Autodesk Inventor part; units mm, degrees
ref_plane "Work Plane2" through (-55.1754, -24.0887, 15.745) normal (0, 0, -1) x (0, 1, 0)
ref_plane "YZ Plane" through (0, 0, 0) normal (1, 0, 0) x (0, 1, 0)
ref_plane "XZ Plane" through (0, 0, 0) normal (0, 1, 0) x (-1, 0, 0)
ref_plane "Work Plane1" through (0, 0, 0) normal (0, 0, 1) x (1, 0, 0)
ref_plane "Work Plane2" through (-55.1754, -24.0887, 15.745) normal (0, 0, -1) x (0, 1, 0)
sketch "Sketch1" plane through (0, 0, 0) normal (0, 0, 1) x (1, 0, 0)
  line L0 (-15.577, -32.8319) -> (-625.177, -32.8319)
  line L1 (-15.577, -13.7819) -> (-625.177, -13.7819)
  line L2 (-51.9475, -0.5269) -> (-51.9475, -17.8187)
  line L3 (-15.577, -10.6107) -> (-15.577, -36.0031)
  line L4 (-51.9475, -45.8894) -> (-31.9475, -45.8894)
  line L5 (-51.9475, -13.7819) -> (-9.7581, -13.7819)
  line L6 (-9.7581, -13.7819) -> (-9.7581, -45.8894)
  line L7 (-9.7581, -45.8894) -> (-51.9475, -45.8894)
  line L8 (-51.9475, -45.8894) -> (-51.9475, -13.7819)
  arc A0 (-55.86, -21.5601) -> (-54.5757, -21.9771) centre (-55.7173, -23.3069) ccw
  arc A1 (-28.9193, -21.5601) -> (-27.635, -21.9771) centre (-28.7766, -23.3069) ccw
  circle A2 centre (-55.7173, -23.3069) radius 1.778
  circle A3 centre (-28.7766, -23.3069) radius 1.778
  circle A4 centre (-37.9475, -17.22) radius 2
  circle A5 centre (-37.9475, -17.22) radius 2
  point P0 (0, 0)
extrude "Extrusion1" add sketch "Sketch1" along normal up to surface (15.745 mm away) contours L3 L5 L6 L7 L4 L8 L0 | L0 L8 L2 L1 L3 | A4
sketch "Sketch2" plane through (-51.9475, -13.7819, 15.745) normal (0, 0, 1) x (1, 0, 0)
  circle A0 centre (6, -26.745) radius 2
  circle A1 centre (14, -26.745) radius 2
  circle A2 centre (6, -26.745) radius 2
  circle A3 centre (14, -26.745) radius 2
  point P0 (51.9475, 13.7819)
hole "Hole1" at (-45.9475, -40.5269, 15.745) direction (0, 0, -1) diameter 3.9878 end through all
sketch "Sketch3" plane through (-51.9475, -13.7819, 15.745) normal (0, 0, 1) x (1, 0, 0)
  circle A0 centre (14, -26.745) radius 2
  circle A1 centre (14, -26.745) radius 2
  point P0 (51.9475, 13.7819)
hole "Hole2" at (-37.9475, -40.5269, 15.745) direction (0, 0, -1) diameter 3.9878 end through all
sketch "Sketch5" plane through (-51.9475, -13.7819, 15.745) normal (0, 0, 1) x (1, 0, 0)
  arc A0 (5.0711, -20.6445) -> (7.8995, -17.8161) centre (6.4853, -19.2303) ccw
  line L0 (4.5858, -20.1592) -> (5.0711, -20.6445)
  arc A1 (7.4142, -17.3308) -> (4.5858, -20.1592) centre (6, -18.745) ccw
  line L1 (7.8995, -17.8161) -> (7.4142, -17.3308)
  arc A2 (7.8995, -3.6739) -> (5.0711, -0.8455) centre (6.4853, -2.2597) ccw
  line L2 (7.4142, -4.1592) -> (7.8995, -3.6739)
  arc A3 (4.5858, -1.3308) -> (7.4142, -4.1592) centre (6, -2.745) ccw
  line L3 (5.0711, -0.8455) -> (4.5858, -1.3308)
  circle A4 centre (6, -26.745) radius 2
  circle A5 centre (14, -26.745) radius 2
  line L4 (20, -4.0368) -> (20, 13.255)
  line L5 (0, 13.255) -> (20, 13.255)
  line L6 (0, 13.255) -> (0, -4.0368)
  arc A6 (0, -17.4532) -> (0, -4.0368) centre (-2, -10.745) ccw
  line L7 (0, -17.4532) -> (0, -32.1075)
  line L8 (0, -32.1075) -> (20, -32.1075)
  line L9 (20, -32.1075) -> (20, -17.4532)
  arc A7 (20, -4.0368) -> (20, -17.4532) centre (22, -10.745) ccw
  circle A8 centre (6, 5.255) radius 2
  circle A9 centre (14, 5.255) radius 2
  arc A10 (12.1005, -17.8161) -> (14.9289, -20.6445) centre (13.5147, -19.2303) ccw
  line L10 (12.5858, -17.3308) -> (12.1005, -17.8161)
  arc A11 (15.4142, -20.1592) -> (12.5858, -17.3308) centre (14, -18.745) ccw
  line L11 (14.9289, -20.6445) -> (15.4142, -20.1592)
  line L12 (10.6863, -8.745) -> (9.3137, -8.745)
  arc A12 (10.6863, -12.745) -> (10.6863, -8.745) centre (10.6863, -10.745) ccw
  line L13 (9.3137, -12.745) -> (10.6863, -12.745)
  arc A13 (9.3137, -8.745) -> (9.3137, -12.745) centre (9.3137, -10.745) ccw
  arc A14 (14.9289, -0.8455) -> (12.1005, -3.6739) centre (13.5147, -2.2597) ccw
  line L14 (15.4142, -1.3308) -> (14.9289, -0.8455)
  arc A15 (12.5858, -4.1592) -> (15.4142, -1.3308) centre (14, -2.745) ccw
  line L15 (12.1005, -3.6739) -> (12.5858, -4.1592)
  line L16 (0, -32.1075) -> (42.1894, -32.1075)
  line L17 (42.1894, 0) -> (0, 0)
  line L18 (42.1894, -32.1075) -> (20, -32.1075)
  line L19 (20, -32.1075) -> (20, 0)
  line L20 (20, 0) -> (42.1894, 0)
  line L21 (42.1894, 0) -> (42.1894, -32.1075)
  point P0 (51.9475, 13.7819)
extrude "Extrusion2" cut sketch "Sketch5" against normal blind 8.0264 contours L4 L17 L21 L16 L9 L19
sketch "Sketch7" plane through (-51.9475, -13.7819, 0) normal (0, 1, 0) x (1, 0, 0)
  line L0 (20, -15.745) -> (20, -7.7186)
  line L1 (0, 0) -> (0, -15.745)
  line L2 (20, -15.745) -> (0, -15.745)
  line L3 (0, -15.745) -> (0, -7.7186)
  line L4 (0, -7.7186) -> (20, -7.7186)
  line L5 (20, -7.7186) -> (20, -15.745)
  point P0 (51.9475, 0)
  dimension "d35" = 8.0264
extrude "Extrusion3" cut sketch "Sketch7" against normal blind 4.445
properties part number "RollerSupport"
Input: part model. Units: mm. Frame: model coordinates. A direction names the side the tool comes from. Give positions to 0.01 mm unless a question says otherwise; leave off trailing zeros. Order: outer loops, then holes, each group sorted by start corner. A loop starts at its lowest first (then second) coordinate and runs counter-clockwise, first axis right, second up. Notation, with made-up numbers: (74, 17) - (131, 17) arc R18 ccw to (131, 27) - close; hole circle Ø2 at (-10, 19.5). An arc over 180 degrees is marked (long way). Answer as a JSON object with one key per item and string values. Group by question number.
Q1. Cut plane D-D, the plane x = -28.5. Output: boundary loops of the cut face in (y, z).
Q2. Cut plane A-A, the plane y = -41.5. Output: boundary loops of the cut face in (x, z) (1 decimal).
Q3. Line query: probe 1 along Y at (x, z) = (-35, 13.25); probe 2 along Z at (x, y) = (-24, -21); probe 3 along Y at (x, z) = (-37.5, 8.75). Output: solid intervals per line, ascending.
Q4. Set-up query: faces 5 (the face through (-42, -18.227, 12)), 6 (the face through (-9.758, -30, 4)), 7 (the face through (-31.948, -32, 12)). Return all of +Z, -Z, +X, -X, +Y, -Y with unobstructed straight access to the full face (end or side cutting, diameter ignored); none if empty.
Q5. First-contact query: pin 1 Ø4 at (x, y) = (-19.5, -37) entering from +Z; pin 2 Ø1 at (y, z) = (-20, 13.5) entering from +X; pin 3 Ø8 at (x, z) = (-37, 13.5) entering from +Y. Flat tips, straight axial feed; report the tip coordinate or a pass-through.
Q6. Cut plane B-B, the plane z = 3.75. Output: boundary loops of the cut face in (x, y), then the cut area to 3 significant figures.
Q7. Mould query, pull axis Y, two halves, no side actions, for faces 1 (the face through (-27.134, -22.626, 3.805)), 2 (the face through (-35, -45.889, 6)), 3 (the face through (-44.18, -41.45, 7.76)), 4 (the face through (-51.948, -30, 8)). Classes: pulls with the +Y half, pulls with the -Y half, needs draft (parallel to the pull), parting line crosses it, or undercut.
Q8. Cut plane C-C, the plane x = -33.5. Output: boundary loops of the cut face in (y, z) (3 decimals).
Results:
{
 "1": {"outline": "(-45.89, 0) - (-25.06, 0) - (-25.06, 7.72) - (-45.89, 7.72) - close; (-21.55, 0) - (-13.78, 0) - (-13.78, 7.72) - (-21.55, 7.72) - close"},
 "2": {"outline": "(-51.9, 0) - (-47.7, 0) - (-47.7, 15.7) - (-51.9, 15.7) - close; (-44.2, 0) - (-39.7, 0) - (-39.7, 15.7) - (-44.2, 15.7) - close; (-36.2, 0) - (-9.8, 0) - (-9.8, 7.7) - (-31.9, 7.7) - (-31.9, 15.7) - (-36.2, 15.7) - close"},
 "3": {"probe 1": "-45.89 to -18.23", "probe 2": "0 to 7.72", "probe 3": "-45.89 to -42.47, -38.58 to -18.23"},
 "4": {"face 5": "+Z, +X, -X, +Y", "face 6": "+Z, -Z, +X, +Y, -Y", "face 7": "+Z, +X, +Y, -Y"},
 "5": {"pin 1": "z = 7.72", "pin 2": "x = -31.95", "pin 3": "y = -18.23"},
 "6": {"outline": "(-51.95, -45.89) - (-9.76, -45.89) - (-9.76, -13.78) - (-51.95, -13.78) - close; hole circle Ø3.99 at (-45.95, -40.53); hole circle Ø3.99 at (-37.95, -40.53); hole circle Ø3.56 at (-28.78, -23.31)", "area": "1,320 mm^2"},
 "7": {"face 1": "undercut", "face 2": "pulls with the -Y half", "face 3": "undercut", "face 4": "needs draft"},
 "8": {"outline": "(-45.889, 0) - (-13.782, 0) - (-13.782, 7.719) - (-18.227, 7.719) - (-18.227, 15.745) - (-45.889, 15.745) - close"}
}
